Here's how the part is built. I have some questions about the finished solid (model axes, mm). A direction names the side the tool comes from. Coordinates: 2 decimals unless noted, no trailing zeros. Loops run counter-clockwise (first coordinate to the right, second up) from the corner with the lowest first, then second, coordinate; pieces in that order, holes last. Notation, with made-up numbers: (8.25, -32) -> (18.25, -32) arc R21 ccw to (18.25, -18) -> close; hole circle Ø5 at (-29.75, 70.25). An arc over 180 degrees is marked (long way). Answer as a JSON object with one key per item and string values. Group by question number.
Q1. I want a section at D-D on y = 17.25. Count the separate pieces of the cut face and the enclosed holes in it, then the cut area to 3 significant figures.
Q2. I want a section at B-B on y = 7.5. Write out the boundary of the cut face in (x, z), then the cut area to 3 significant figures.
Q3. Thinking about a two-plate mould opening in Y: for faces 6 (the flat face through (48, -2, 10)), 7 (the flat face through (5.767, 17.718, 10.14)), 8 (the cylindrical face through (29, -3.5, 9.1)), 9 (the cylindrical face through (87.07, 0.916, -10.315)), which applies, released by +Y, released by -Y, zero draft, split by the parting line, or undercut?
Q4. I need wall thicknesses on line 1 (X direction, y = -3.05, z = 10); line 2 (Y direction, x = 87.75, z = -12.6); line 3 (Y direction, x = 84, z = 18). Which ranges of each line are inside material? Lowest first, please.
Q5. On a 3-axis mill with a long thin cutter (end or side, diameter ignored), from which of +Z, -Z, +X, -X, +Y, -Y can I reach the whole of each face in a straight line? I mean faces 1 (the flat face through (40.49, 17.78, 10.14)), 2 (the flat face through (2, 15.5, 10)), 3 (the cylindrical face through (45.79, -3.52, 10.38)), 4 (the flat face through (82, 5, 39)), 5 (the flat face through (0, 5, 10)). Say none if no direction works.
Q6. I want a section at C-C on z = -21. Write out the boundary of the cut face in (x, y).
Q7. I'm going to push flat-ended pins straight in: pin 1 (4 mm diameter, centred on x = 55.5, y = 12.5, fed in from -Z); pin 2 (1 mm diameter, centred on x = 46.5, z = 9.5, fed in from -Y); pin 3 (9.5 mm diameter, centred on x = 80, z = 9.5, fed in from +Y). Where does each tip first touch, or does it pass through?
Q8. I want a section at A-A on z = 32.6. Write out the boundary of the cut face in (x, y), then the cut area to 3 significant figures.
```python
from build123d import *

# Parameters (mm, degrees)
SKETCH_1_W             = 92
SKETCH_1_H             = 20
EXTRUDE_1_DEPTH        = 20
CUT_EXTRUDE_1_DEPTH    = 97.249675324
PATTERN_LINEAR_1_COUNT = 14
PATTERN_LINEAR_1_PITCH = 6.28
CUT_EXTRUDE_2_DEPTH    = 97.249675324
SKETCH_4_W             = 30
SKETCH_4_H             = 15.5
EXTRUDE_2_DEPTH        = 10
EXTRUDE_3_DEPTH        = 5
SKETCH_9_R             = 4.25
CUT_EXTRUDE_6_DEPTH    = 107.60206377
SKETCH_11_W            = 20
SKETCH_11_H            = 5
EXTRUDE_4_DEPTH        = 82
SKETCH_12_R            = 1.75
CUT_EXTRUDE_7_DEPTH    = 3


with BuildPart() as part:
    # 草图1 → 凸台-拉伸1 (new body)
    with BuildSketch(Plane.XY):
        with Locations((46, 10)):
            Rectangle(SKETCH_1_W, SKETCH_1_H)
    extrude(amount=EXTRUDE_1_DEPTH)

    # 草图2 → 切除-拉伸1 (cut, through all)
    with BuildSketch(Plane.XY.offset(20)):
        Polygon((2, 20), (3.637866054, 15.5), (4.959614883, 15.5), (6.597480937, 20), align=None)
    cut_extrude_1 = extrude(amount=-CUT_EXTRUDE_1_DEPTH, mode=Mode.SUBTRACT)

    # 阵列(线性)1: 切除-拉伸1 ×14
    with Locations(*[(i * PATTERN_LINEAR_1_PITCH, 0, 0) for i in range(1, PATTERN_LINEAR_1_COUNT)]):
        add(cut_extrude_1, mode=Mode.SUBTRACT)

    # 草图3 → 切除-拉伸2 (cut, through all)
    with BuildSketch(Plane.XY.offset(20)):
        Polygon((2, 20), (0, 20), (0, 15.5), (3.637866054, 15.5), align=None)
        Polygon((74.039614883, 15.5), (75.677480937, 20), (92, 20), (92, 15.5), align=None)
    extrude(amount=-CUT_EXTRUDE_2_DEPTH, mode=Mode.SUBTRACT)

    # 草图4 → 凸台-拉伸2 (add)
    with BuildSketch(Plane(origin=(92, 0, 0), x_dir=(0, 0, -1), z_dir=(1, 0, 0))):
        with Locations((-35, 7.75)):
            Rectangle(SKETCH_4_W, SKETCH_4_H)
        with Locations((15, 7.75)):
            Rectangle(SKETCH_4_W, SKETCH_4_H)
    extrude(amount=-EXTRUDE_2_DEPTH)

    # 草图6 → 凸台-拉伸3 (add)
    with BuildSketch(Plane.XZ):
        Polygon((82, 0), (82, 20), (82, 50), (92, 50), (92, -30), (82, -30), align=None)
    extrude(amount=EXTRUDE_3_DEPTH)

    # 草图9 → 切除-拉伸6 (cut, through all)
    with BuildSketch(Plane(origin=(92, 0, 0), x_dir=(0, 0, -1), z_dir=(1, 0, 0))):
        with Locations((-32.6, 4.5)):
            Circle(SKETCH_9_R)
        with Locations(Location((12.6, 4.5, 0), (0, 0, 180))):
            Circle(SKETCH_9_R)
    extrude(amount=-CUT_EXTRUDE_6_DEPTH, mode=Mode.SUBTRACT)

    # 草图11 → 凸台-拉伸4 (add)
    with BuildSketch(Plane.ZY):
        with Locations((10, -2.5)):
            Rectangle(SKETCH_11_W, SKETCH_11_H)
    extrude(amount=-EXTRUDE_4_DEPTH)

    # 草图12 → 切除-拉伸7 (cut)
    with BuildSketch(Plane.XZ.offset(5)):
        with Locations(Location((7.5, 10, 0), (0, 0, 270))):
            Circle(SKETCH_12_R)
        with Locations(Location((27.5, 10, 0), (0, 0, 270))):
            Circle(SKETCH_12_R)
        with Locations(Location((47.5, 10, 0), (0, 0, 270))):
            Circle(SKETCH_12_R)
    extrude(amount=-CUT_EXTRUDE_7_DEPTH, mode=Mode.SUBTRACT)


solid = part.part
```
Result set:
{
 "1": {"separate pieces": "11", "enclosed holes": "0", "area": "811 mm²"},
 "2": {"outline": "(0, 0) -> (82, 0) -> (82, -9.59) -> (92, -9.59) -> (92, 29.59) -> (82, 29.59) -> (82, 20) -> (0, 20) -> close; (82, -30) -> (92, -30) -> (92, -15.61) -> (82, -15.61) -> close; (82, 35.61) -> (92, 35.61) -> (92, 50) -> (82, 50) -> close", "area": "2,320 mm²"},
 "3": {"face 6": "released by -Y", "face 7": "released by +Y", "face 8": "zero draft", "face 9": "undercut"},
 "4": {"line 1": "x = 0 to 5.75, 9.25 to 25.75, 29.25 to 45.75, 49.25 to 92", "line 2": "y = -5 to 0.25, 8.75 to 15.5", "line 3": "y = -5 to 15.5"},
 "5": {"face 1": "+Z, -Z, +Y", "face 2": "+Z, -Z, -X, +Y", "face 3": "-Y", "face 4": "+Z, -X, +Y, -Y", "face 5": "+Z, -Z, -X, +Y, -Y"},
 "6": {"outline": "(82, -5) -> (92, -5) -> (92, 15.5) -> (82, 15.5) -> close"},
 "7": {"pin 1": "stops at z = 0", "pin 2": "stops at y = -2", "pin 3": "stops at y = 15.5"},
 "8": {"outline": "(82, -5) -> (92, -5) -> (92, 0.25) -> (82, 0.25) -> close; (82, 8.75) -> (92, 8.75) -> (92, 15.5) -> (82, 15.5) -> close", "area": "120 mm²"}
}
